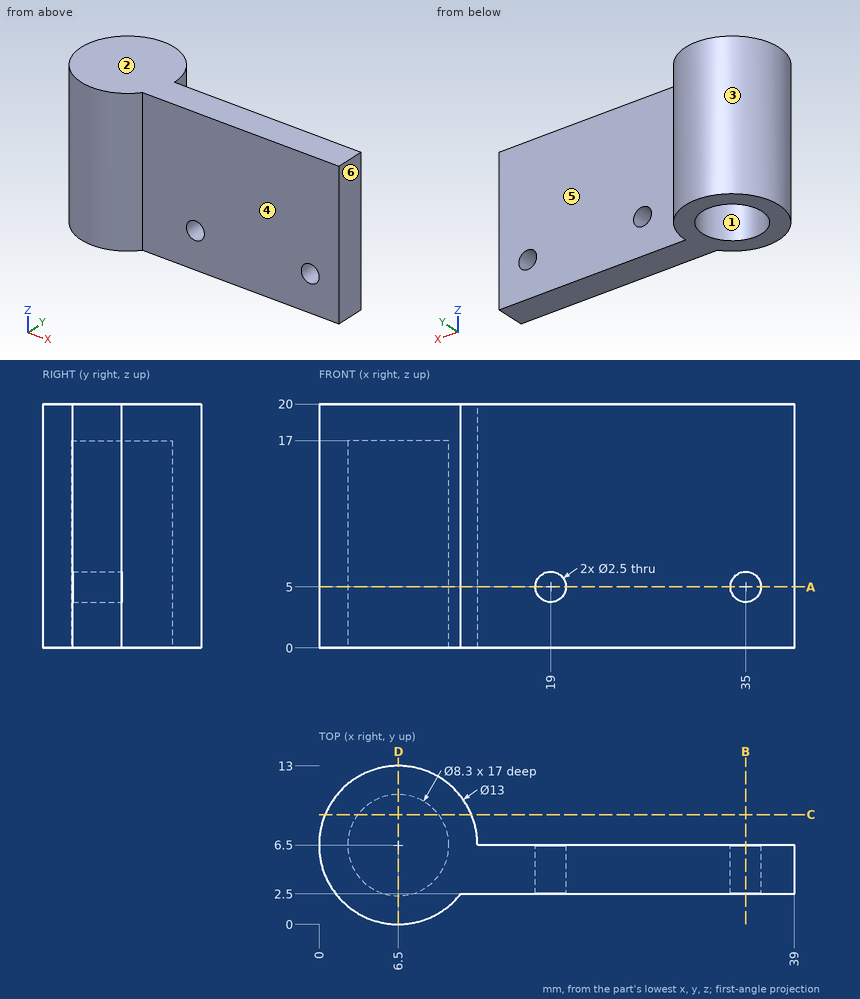
For this review, use the dimensioned drawing (mm, ordinates from the lowest corner) and the shaded views. A direction names the side the tool comes from. Round coordinates to 2 decimals unless told otherwise and drop trailing zeros. Order: outer loops, then holes, each group sorted by start corner. A loop starts at its lowest first (then second) coordinate and runs counter-clockwise, first axis right, second up.
1) Clearance check with flat-ended pins moving along their axes: pin 1 Ø7.5 at (x, y) = (6.5, 6.5) entering from -Z; pin 2 Ø10 at (x, z) = (22, 6) entering from -Y; pin 3 Ø1.5 at (x, z) = (11, 4.5) entering from -Y. State where each tip first meets the part, or that it passes through.
The answers:
pin 1: stops at z = 17
pin 2: stops at y = 2.5
pin 3: stops at y = 1.19
2) Consider section C-C (y = 9). State the section outline as (x, z) points.
The answers:
outline: (0.5, 0) - (3.19, 0) - (3.19, 17) - (9.81, 17) - (9.81, 0) - (12.5, 0) - (12.5, 20) - (0.5, 20) - close
3) Consider section D-D (x = 6.5). State the section outline as (y, z) points.
The answers:
outline: (0, 0) - (2.35, 0) - (2.35, 17) - (10.65, 17) - (10.65, 0) - (13, 0) - (13, 20) - (0, 20) - close
4) Draft analysis for pull direction Y (two halves, no side actions). For the marked faces 1, 2 and 3, state which applies: released by +Y, released by -Y, zero draft, split by the parting line, or undercut.
The answers:
face 1: undercut
face 2: zero draft
face 3: split by the parting line
5) For L1, parallel to Z at x = 19, y = 5.5; L2, parallel to X at y = 4.85, z = 5; L3, parallel to Y at x = 6.5, z = 6.75, list the stretches that pass through material, from the lowest coordinate up.
The answers:
L1: z = 0 to 3.75, 6.25 to 20
L2: x = 0.21 to 2.69, 10.31 to 17.75, 20.25 to 33.75, 36.25 to 39
L3: y = 0 to 2.35, 10.65 to 13
6) Machinability: for the marked faces 4, 5 and 6, which of the approach directions +Z, -Z, +X, -X, +Y, -Y give a long, thin tool a straight path to every point of the face, cutting with its end or side? Answer none if there is none.
The answers:
face 4: +Z, -Z, +X, -Y
face 5: +Z, -Z, +X, +Y
face 6: +Z, -Z, +X, +Y, -Y
7) Consider section B-B (x = 35). State the section outline as (y, z) points.
The answers:
outline: (2.5, 0) - (6.5, 0) - (6.5, 3.75) - (2.5, 3.75) - close; (2.5, 6.25) - (6.5, 6.25) - (6.5, 20) - (2.5, 20) - close
8) Consider section A-A (z = 5). State the section outline as (x, y) points, plus the area to 3 significant figures.
The answers:
outline: (11.62, 2.5) - (17.75, 2.5) - (17.75, 6.5) - (13, 6.5) arc R6.5 ccw (long way) to start; (20.25, 2.5) - (33.75, 2.5) - (33.75, 6.5) - (20.25, 6.5) - close; (36.25, 2.5) - (39, 2.5) - (39, 6.5) - (36.25, 6.5) - close; hole circle Ø8.3 at (6.5, 6.5)
area: 164 mm2
